For this review, take the finished solid that the model builds, in its own axes (mm). Face numbers are marked on the shaded views. A direction names the side the tool comes from. Coordinates: 2 decimals unless noted, no trailing zeros. Loops run counter-clockwise (first coordinate to the right, second up) from the corner with the lowest first, then second, coordinate; pieces in that order, holes last. Notation, with made-up numbers: (36.5, 47.5) - (75.5, 47.5) arc R16 cw to (75.5, 57.5) - close; hole circle Ø9 at (27.25, -39.75). An arc over 180 degrees is marked (long way). One line per item, written item: value. Start each with the question number.
1. Take a section at D-D, the plane x = -13.5. State the section outline as (y, z) points (1 decimal), and give its area (3 significant figures).
2. Take a section at B-B, the plane x = -4.5. State the section outline as (y, z) points (1 decimal), and give its area (3 significant figures).
3. Insertion check: pin 1 (1.3 mm diameter, centred on x = -31.5, z = 7, fed in from +Y); pin 2 (2.5 mm diameter, centred on y = -3.5, z = 1.5, fed in from -X); pin 3 (1.7 mm diameter, centred on x = -13, z = 6.5, fed in from +Y); pin 4 (1.5 mm diameter, centred on y = -8, z = 2, fed in from +X). Each pin has a flat end and moves straight along its axis. Give the tip position at first contact, or say it passes through.
4. The part is to be moulded in two halves that separate along X. For the marked faces 4, 5, 6 and 7, say which applies: released by +X, released by -X, zero draft, split by the parting line, or undercut.
5. To check wall thickness, follow line 1 (Y direction, x = -21, z = 3.75); line 2 (X direction, y = -5.5, z = 1); line 3 (X direction, y = -4.75, z = 1). State the ranges of each line that lie inside material, in increasing order. Write a range as from..to.
6. Take a section at A-A, the plane z = 2.5. State the section outline as (x, y) points.
7. Take a section at C-C, the plane y = -1. State the section outline as (x, z) points, and give its area (3 significant figures).
8. For the marked faces 1, 2 and 3, list the 3-axis set-ups (+Z, -Z, +X, -X, +Y, -Y) from which the entire face can be reached by the end or side of a thin tool; tool diameter is ignored.
```python
from build123d import *

# Parameters (mm, degrees)
SKETCH1_W                       = 73
SKETCH1_H                       = 7.715
BOSS_EXTRUDE1_DEPTH             = 8.5
BOSS_EXTRUDE5_REACH             = 40.165
BOSS_EXTRUDE5_DIRECTION_2_REACH = 40.165
SKETCH6_W                       = 12
SKETCH6_H                       = 3.715
CUT_EXTRUDE1_DEPTH              = 9
SKETCH7_R                       = 1.5875
CUT_EXTRUDE2_DEPTH              = 2.5
CUT_EXTRUDE3_DEPTH              = 2.54
BOSS_EXTRUDE6_DEPTH             = 2.54


with BuildPart() as part:
    # Sketch1 → Boss-Extrude1 (new body)
    with BuildSketch(Plane(origin=(0, 0, 0), x_dir=(1, 0, 0), z_dir=(0, 1, 0))):
        with Locations((0, -3.3575)):
            Rectangle(SKETCH1_W, SKETCH1_H)
    extrude(amount=BOSS_EXTRUDE1_DEPTH)

    # Boss-Extrude5: up to this face of the body (flat: up to its plane)
    boss_extrude5_end = Plane(part.part.faces().sort_by_distance((0, 4.25, 7.215))[0])
    # Sketch5 → Boss-Extrude5 (add, up to the picked face)
    with BuildSketch(Plane.XY, mode=Mode.PRIVATE) as boss_extrude5_sk1:
        with BuildLine():
            Line((-2.54, -6), (-2.54, -9))
            Line((-2.54, -9), (-6, -9))
            Line((-6, -9), (-6, 0))
            Line((-6, 0), (6, 0))
            Line((6, 0), (6, -9))
            Line((6, -9), (2.54, -9))
            Line((2.54, -9), (2.54, -6))
            ThreePointArc((2.54, -6), (0, -3.46), (-2.54, -6))
        make_face()
    boss_extrude5_tool1 = split(extrude(boss_extrude5_sk1.sketch, amount=BOSS_EXTRUDE5_REACH, mode=Mode.PRIVATE), bisect_by=boss_extrude5_end, keep=Keep.BOTH, mode=Mode.PRIVATE)
    add(boss_extrude5_tool1.solids().sort_by(Axis((-2.69, -7.5, 0), (0, 0, 1)))[0])

    # Boss-Extrude5 direction 2: up to this face of the body (flat: up to its plane)
    boss_extrude5_direction_2_end = Plane(part.part.faces().sort_by_distance((0, 4.25, -0.5))[0])
    # Sketch5 → Boss-Extrude5 direction 2 (add, up to the picked face)
    with BuildSketch(Plane.XY, mode=Mode.PRIVATE) as boss_extrude5_direction_2_sk1:
        with BuildLine():
            Line((-2.54, -6), (-2.54, -9))
            Line((-2.54, -9), (-6, -9))
            Line((-6, -9), (-6, 0))
            Line((-6, 0), (6, 0))
            Line((6, 0), (6, -9))
            Line((6, -9), (2.54, -9))
            Line((2.54, -9), (2.54, -6))
            ThreePointArc((2.54, -6), (0, -3.46), (-2.54, -6))
        make_face()
    boss_extrude5_direction_2_tool1 = split(extrude(boss_extrude5_direction_2_sk1.sketch, amount=-BOSS_EXTRUDE5_DIRECTION_2_REACH, mode=Mode.PRIVATE), bisect_by=boss_extrude5_direction_2_end, keep=Keep.BOTH, mode=Mode.PRIVATE)
    add(boss_extrude5_direction_2_tool1.solids().sort_by(Axis((-2.69, -7.5, 0), (0, 0, -1)))[0])

    # Sketch6 → Cut-Extrude1 (cut)
    with BuildSketch(Plane.XZ.offset(9)):
        with Locations((0, 3.3575)):
            Rectangle(SKETCH6_W, SKETCH6_H)
    extrude(amount=-CUT_EXTRUDE1_DEPTH, mode=Mode.SUBTRACT)

    # Sketch7 → Cut-Extrude2 (cut)
    with BuildSketch(Plane(origin=(0, 8.5, 0), x_dir=(1, 0, 0), z_dir=(0, 1, 0))):
        with Locations((0, -7.215)):
            Circle(SKETCH7_R)
        with Locations((4.5, -7.215)):
            Circle(SKETCH7_R)
        with Locations((9, -7.215)):
            Circle(SKETCH7_R)
        with Locations((13.5, -7.215)):
            Circle(SKETCH7_R)
        with Locations((18, -7.215)):
            Circle(SKETCH7_R)
        with Locations((22.5, -7.215)):
            Circle(SKETCH7_R)
        with Locations((27, -7.215)):
            Circle(SKETCH7_R)
        with Locations((31.5, -7.215)):
            Circle(SKETCH7_R)
        with Locations((-31.5, -7.215)):
            Circle(SKETCH7_R)
        with Locations((-27, -7.215)):
            Circle(SKETCH7_R)
        with Locations((-22.5, -7.215)):
            Circle(SKETCH7_R)
        with Locations((-18, -7.215)):
            Circle(SKETCH7_R)
        with Locations((-13.5, -7.215)):
            Circle(SKETCH7_R)
        with Locations((-9, -7.215)):
            Circle(SKETCH7_R)
        with Locations((-4.5, -7.215)):
            Circle(SKETCH7_R)
        with BuildLine():
            Line((36, -5.6275), (36.5, -5.6275))
            Line((36.5, -5.6275), (36.5, -5.70829623))
            ThreePointArc((36.5, -5.70829623), (35.746757018, -8.782170776), (36, -5.6275))
        make_face()
        with BuildLine():
            Line((-36.5, -5.6275), (-36.5, -5.70829623))
            ThreePointArc((-36.5, -5.70829623), (-35.746757018, -8.782170776), (-36, -5.6275))
            Line((-36, -5.6275), (-36.5, -5.6275))
        make_face()
    extrude(amount=-CUT_EXTRUDE2_DEPTH, mode=Mode.SUBTRACT)

    # Sketch8 → Cut-Extrude3 (cut)
    with BuildSketch(Plane(origin=(0, 0, 5.215), x_dir=(-1, 0, 0), z_dir=(0, 0, -1))):
        with BuildLine():
            Line((2.54, -6), (2.54, -9))
            Line((2.54, -9), (6, -9))
            Line((6, -9), (6, 0))
            Line((6, 0), (-6, 0))
            Line((-6, 0), (-6, -9))
            Line((-6, -9), (-2.54, -9))
            Line((-2.54, -9), (-2.54, -6))
            ThreePointArc((-2.54, -6), (0, -3.46), (2.54, -6))
        make_face()
    extrude(amount=-CUT_EXTRUDE3_DEPTH, mode=Mode.SUBTRACT)

    # Sketch9 → Boss-Extrude6 (add)
    with BuildSketch(Plane.XY.offset(1.5)):
        with BuildLine():
            Line((2.54, -9), (6, -9))
            Line((6, -9), (6, 0))
            Line((6, 0), (-6, 0))
            Line((-6, 0), (-6, -9))
            Line((-6, -9), (-2.54, -9))
            Line((-2.54, -9), (-2.54, -6))
            ThreePointArc((-2.54, -6), (0, -3.46), (2.54, -6))
            Line((2.54, -6), (2.54, -9))
        make_face()
    extrude(amount=BOSS_EXTRUDE6_DEPTH)


solid = part.part
```
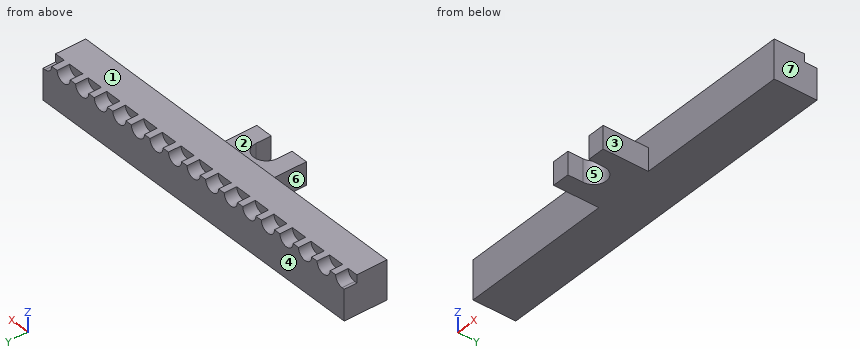
Solutions:
1. outline: (0, -0.5) - (8.5, -0.5) - (8.5, 5.6) - (6, 5.6) - (6, 7.2) - (0, 7.2) - close
1. area: 61.6 mm2
2. outline: (-9, -0.5) - (8.5, -0.5) - (8.5, 5.6) - (6, 5.6) - (6, 7.2) - (0, 7.2) - (0, 4) - (-9, 4) - close
2. area: 102 mm2
3. pin 1: y = 6
3. pin 2: x = -6
3. pin 3: y = 8.5
3. pin 4: x = 6
4. face 4: zero draft
4. face 5: undercut
4. face 6: released by -X
4. face 7: released by +X
5. line 1: 0..8.5
5. line 2: -6..-2.49, 2.49..6
5. line 3: -6..-2.21, 2.21..6
6. outline: (-36.5, 0) - (-6, 0) - (-6, -9) - (-2.54, -9) - (-2.54, -6) arc R2.54 cw to (2.54, -6) - (2.54, -9) - (6, -9) - (6, 0) - (36.5, 0) - (36.5, 8.5) - (-36.5, 8.5) - close
7. outline: (-6, -0.5) - (6, -0.5) - (6, 4.04) - (-6, 4.04) - close
7. area: 54.5 mm2
8. face 1: +Z, +X, -X, +Y, -Y
8. face 2: +Z, +X, -X, -Y
8. face 3: +Z, -Z, +X, -Y
